Check sheet for the modelled part. Datum: model origin and axes. Units: mm. Face numbers are marked on the shaded views. Coordinates: 2 decimals unless noted, no trailing zeros. Order: outer loops, then holes, each group sorted by start corner. A loop starts at its lowest first (then second) coordinate and runs counter-clockwise, first axis right, second up.
1. Cross-section at C-C (x = -15). Enter the section's corners in (y, z), then the cut area to 3 significant figures.
2. Cross-section at A-A (z = 5). Enter the section's corners in (x, y).
3. Draft check along Y on the marked faces 1 and 2. Enter one of: released by +Y, released by -Y, zero draft, split by the parting line, or undercut.
4. Thickness scan on line 1 (X direction, y = -7, z = 5.55); line 2 (Z direction, x = -5.5, y = 22); line 3 (X direction, y = -17, z = 4.4). Record the ranges inside material, lowest first.
5. Cross-section at B-B (y = -12). Enter the section's corners in (x, z), then the cut area to 3 significant figures.
6. Gauge pin test, flat ends, axial feed: pin 1 Ø3 at (x, z) = (-31.5, 5) entering from -Y; pin 2 Ø8 at (x, y) = (9, 30.5) entering from -Z; pin 3 Ø2 at (x, z) = (-26.5, 5) entering from +Y; pin 4 Ø3 at (x, y) = (-38, 31) entering from +Z. Record the tip position at first contact, or that the pin passes through.
7. Cross-section at D-D (x = -38.5). Enter the section's corners in (y, z).
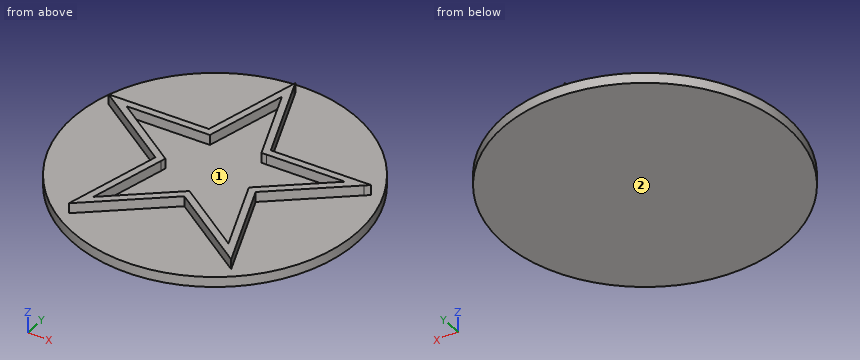
```python
from build123d import *

# Parameters (mm, degrees)
F1_DEPTH = 6
F0_R     = 41.694861
F2_DEPTH = 3


with BuildPart() as f1:
    # F0 (on Top) → F1 (new body)
    with BuildSketch(Plane.XY):
        Polygon((-18.393972, 19.060652), (-46.477814, 17.770472), (-22.999159, 2.306981), (-30.450509, -24.801028), (-8.488552, -7.249981), (14.990103, -22.713471), (5.084683, 3.597162), (25.7176, 20.086097), (27.04664, 21.148209), (-1.037203, 19.858028), (-10.34319, 44.576459), (-10.942622, 46.168661), align=None)
        Polygon((10.949591, -17.657503), (-7.388475, -5.579703), (-8.602003, -4.78045), (-9.737139, -5.687601), (-26.890584, -19.395893), (-21.070687, 1.77689), (-20.685553, 3.178007), (-40.237148, 16.05506), (-16.850634, 17.129444), (-10.645603, 39.703344), (-2.396973, 17.79345), (-0.945419, 17.860135), (20.989542, 18.867834), (2.700961, 4.252391), (3.212937, 2.892488), align=None, mode=Mode.SUBTRACT)
    extrude(amount=F1_DEPTH)

    # F0 (on Top) → F2 (join)
    with BuildSketch(Plane.XY):
        with Locations((-9.16684, 7.514569)):
            Circle(F0_R)
        Polygon((-22.999159, 2.306981), (-46.477814, 17.770472), (-18.393972, 19.060652), (-10.942622, 46.168661), (-10.34319, 44.576459), (-1.037203, 19.858028), (27.04664, 21.148209), (25.7176, 20.086097), (5.084683, 3.597162), (14.990103, -22.713471), (-8.488552, -7.249981), (-30.450509, -24.801028), align=None, mode=Mode.SUBTRACT)
        Polygon((-8.602003, -4.78045), (-7.388475, -5.579703), (10.949591, -17.657503), (3.212937, 2.892488), (2.700961, 4.252391), (20.989542, 18.867834), (-0.945419, 17.860135), (-2.396973, 17.79345), (-10.645603, 39.703344), (-16.850634, 17.129444), (-40.237148, 16.05506), (-20.685553, 3.178007), (-21.070687, 1.77689), (-26.890584, -19.395893), (-9.737139, -5.687601), align=None)
    extrude(amount=F2_DEPTH)


solid = f1.part
```
Data:
1. outline: (-33.77, 0) - (48.8, 0) - (48.8, 3) - (31.41, 3) - (31.41, 6) - (23.86, 6) - (23.86, 3) - (-9.89, 3) - (-9.89, 6) - (-12.45, 6) - (-12.45, 3) - (-33.77, 3) - close
1. area: 278 mm2
2. outline: (-46.48, 17.77) - (-23, 2.31) - (-30.45, -24.8) - (-8.49, -7.25) - (14.99, -22.71) - (5.08, 3.6) - (25.72, 20.09) - (27.05, 21.15) - (-1.04, 19.86) - (-10.34, 44.58) - (-10.94, 46.17) - (-18.39, 19.06) - close; hole (-40.24, 16.06) - (-20.69, 3.18) - (-26.89, -19.4) - (-9.74, -5.69) - (-8.6, -4.78) - (-7.39, -5.58) - (10.95, -17.66) - (3.21, 2.89) - (2.7, 4.25) - (20.99, 18.87) - (-0.95, 17.86) - (-2.4, 17.79) - (-10.65, 39.7) - (-16.85, 17.13) - close
3. face 1: undercut
3. face 2: zero draft
4. line 1: x = -25.56 to -23.48, -11.38 to -5.23, 6.94 to 9.07
4. line 2: z = 0 to 3
4. line 3: x = -28.31 to -26.23, -23.89 to -20.69, 6.32 to 9.95, 10.7 to 12.84
5. outline: (-46.01, 0) - (27.68, 0) - (27.68, 3) - (10.96, 3) - (10.96, 6) - (8.82, 6) - (8.82, 3) - (2.36, 3) - (2.36, 6) - (-1.28, 6) - (-1.28, 3) - (-14.43, 3) - (-14.43, 6) - (-17.64, 6) - (-17.64, 3) - (-24.86, 3) - (-24.86, 6) - (-26.93, 6) - (-26.93, 3) - (-46.01, 3) - close
5. area: 254 mm2
6. pin 1: stops at y = -24.8
6. pin 2: stops at z = 0
6. pin 3: stops at y = 18.73
6. pin 4: stops at z = 3
7. outline: (-22.12, 0) - (37.15, 0) - (37.15, 3) - (18.14, 3) - (18.14, 6) - (16.13, 6) - (16.13, 3) - (14.91, 3) - (14.91, 6) - (12.52, 6) - (12.52, 3) - (-22.12, 3) - close
